Read the model definition and answer for the solid it produces. Units are mm, in the model's axes. Face numbers are marked on the shaded views. A direction names the side the tool comes from. Coordinates: 2 decimals unless noted, no trailing zeros. Order: outer loops, then holes, each group sorted by start corner. A loop starts at its lowest first (then second) coordinate and runs counter-clockwise, first axis right, second up.
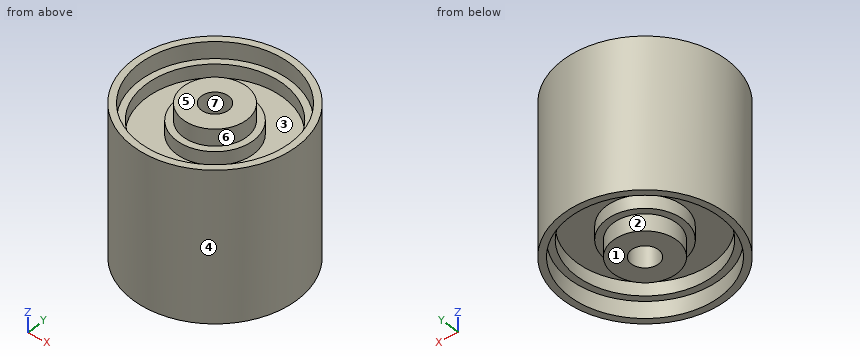
from build123d import *

# Parameters (mm, degrees)
SKETCH1_R           = 24.5
SKETCH1_R_2         = 4.05
BOSS_EXTRUDE1_DEPTH = 45
SKETCH2_R           = 20.5
SKETCH2_R_2         = 11.5
CUT_EXTRUDE1_DEPTH  = 9
CUT_EXTRUDE2_START  = -9
SKETCH3_R           = 20.5
SKETCH3_R_2         = 11.5
CUT_EXTRUDE2_DEPTH  = 9
SKETCH5_R           = 22.5
SKETCH5_R_2         = 9.5
CUT_EXTRUDE3_DEPTH  = 5
CUT_EXTRUDE4_START  = -5
SKETCH6_R           = 22.5
SKETCH6_R_2         = 9.5
CUT_EXTRUDE4_DEPTH  = 5


with BuildPart() as part:
    # Sketch1 → Boss-Extrude1 (new body)
    with BuildSketch(Plane.XY):
        Circle(SKETCH1_R)
        Circle(SKETCH1_R_2, mode=Mode.SUBTRACT)
    extrude(amount=-BOSS_EXTRUDE1_DEPTH)

    # Sketch2 → Cut-Extrude1 (cut)
    with BuildSketch(Plane.XY):
        Circle(SKETCH2_R)
        Circle(SKETCH2_R_2, mode=Mode.SUBTRACT)
    extrude(amount=-CUT_EXTRUDE1_DEPTH, mode=Mode.SUBTRACT)

    # Sketch3 → Cut-Extrude2 (cut)
    with BuildSketch(Plane(origin=(0, 0, -45), x_dir=(-1, 0, 0), z_dir=(0, 0, -1)).offset(CUT_EXTRUDE2_START)):
        with Locations(Location((0, 0, 0), (0, 0, 180))):
            Circle(SKETCH3_R)
        with Locations(Location((0, 0, 0), (0, 0, 180))):
            Circle(SKETCH3_R_2, mode=Mode.SUBTRACT)
    extrude(amount=CUT_EXTRUDE2_DEPTH, mode=Mode.SUBTRACT)

    # Sketch5 → Cut-Extrude3 (cut)
    with BuildSketch(Plane.XY):
        Circle(SKETCH5_R)
        Circle(SKETCH5_R_2, mode=Mode.SUBTRACT)
    extrude(amount=-CUT_EXTRUDE3_DEPTH, mode=Mode.SUBTRACT)

    # Sketch6 → Cut-Extrude4 (cut)
    with BuildSketch(Plane(origin=(0, 0, -45), x_dir=(-1, 0, 0), z_dir=(0, 0, -1)).offset(CUT_EXTRUDE4_START)):
        with Locations(Location((0, 0, 0), (0, 0, 180))):
            Circle(SKETCH6_R)
        with Locations(Location((0, 0, 0), (0, 0, 180))):
            Circle(SKETCH6_R_2, mode=Mode.SUBTRACT)
    extrude(amount=CUT_EXTRUDE4_DEPTH, mode=Mode.SUBTRACT)


solid = part.part
Q1. Which of the six approach directions +Z, -Z, +X, -X, +Y, -Y give full straight-line access (tool end or side, diameter ignored) to the marked faces 1, 2 and 3?
Q2. The part is cut by section A-A, the plane z = -21.5. Determine the outline of the cut face in (x, y).
Q3. The part is cut by section C-C, the plane x = -14.5. Determine the outline of the cut face in (y, z), then the cut area to 3 significant figures.
Q4. Straight lines are drawn through the part: L1, parallel to Y at x = 0, z = -42.9; L2, parallel to Y at x = 0, z = -38.1; L3, parallel to Y at x = 9, z = -37. For each, find the intervals that lie inside material, in ascending order.
Q5. Each of these flat-tipped pins is pushed along its axis until it touches: P1, Ø2, axis at y = -18, z = -36.5, coming from the +X side; P2, Ø6, axis at x = -13, y = 6, coming from the +Z side; P3, Ø1.5, axis at x = -5.5, y = 14.5, coming from the -Z side; P4, Ø7.5, axis at x = 0, y = 0, coming from the -Z side. Where does it stop, or does it pass through?
Q6. The part is cut by section B-B, the plane y = -19. Determine the outline of the cut face in (x, z).
Q7. Determine the mould class of the marked faces 4, 5, 6 and 7 for opening direction X: +X half, -X half, draft (parallel to the pull), parting line (faces both ways), or undercut.
Computed values:
1. face 1: -Z, +X, -X, +Y, -Y
1. face 2: -Z
1. face 3: +Z
2. outline: circle Ø49 at (0, 0); hole circle Ø8.1 at (0, 0)
3. outline: (-19.75, -45) - (-17.2, -45) - (-17.2, -40) - (-14.49, -40) - (-14.49, -36) - (14.49, -36) - (14.49, -40) - (17.2, -40) - (17.2, -45) - (19.75, -45) - (19.75, 0) - (17.2, 0) - (17.2, -5) - (14.49, -5) - (14.49, -9) - (-14.49, -9) - (-14.49, -5) - (-17.2, -5) - (-17.2, 0) - (-19.75, 0) - close
3. area: 1,200 mm2
4. L1: y = -24.5 to -22.5, -9.5 to -4.05, 4.05 to 9.5, 22.5 to 24.5
4. L2: y = -24.5 to -20.5, -11.5 to -4.05, 4.05 to 11.5, 20.5 to 24.5
4. L3: y = -22.79 to -18.42, -7.16 to 7.16, 18.42 to 22.79
5. P1: stops at x = 17.64
5. P2: stops at z = -5
5. P3: stops at z = -36
5. P4: passes through
6. outline: (-15.47, -45) - (-12.05, -45) - (-12.05, -40) - (-7.7, -40) - (-7.7, -36) - (7.7, -36) - (7.7, -40) - (12.05, -40) - (12.05, -45) - (15.47, -45) - (15.47, 0) - (12.05, 0) - (12.05, -5) - (7.7, -5) - (7.7, -9) - (-7.7, -9) - (-7.7, -5) - (-12.05, -5) - (-12.05, 0) - (-15.47, 0) - close
7. face 4: parting line
7. face 5: draft
7. face 6: undercut
7. face 7: undercut
